Geometry check sheet. Reference: the model listing, model coordinates, mm. A direction names the side the tool comes from. Coordinates: 2 decimals unless noted, no trailing zeros. Loops run counter-clockwise (first coordinate to the right, second up) from the corner with the lowest first, then second, coordinate; pieces in that order, holes last. Notation, with made-up numbers: M -28,-32.75 L -15,-32.75 A17 cw -15,-9.75 Z; hole C 43.25,17 d5. An arc over 180 degrees is marked long. One line per question, with ' | ' between items. Start each with the question number.
from build123d import *

# Parameters (mm, degrees)
SKETCH1_R           = 3.625
SKETCH1_R_2         = 2.075
BOSS_EXTRUDE1_DEPTH = 2.41
SKETCH2_R           = 1
SKETCH2_R_2         = 0.5
BOSS_EXTRUDE3_DEPTH = 1.89
BOSS_EXTRUDE4_START = 4.3
SKETCH1_2_R         = 3.625
SKETCH1_2_R_2       = 2.075
BOSS_EXTRUDE4_DEPTH = 0.8
SKETCH3_R           = 1.5875
CUT_EXTRUDE1_DEPTH  = 18.958844524


with BuildPart() as part:
    # Sketch1 → Boss-Extrude1 (new body)
    with BuildSketch(Plane(origin=(0, 0, 0), x_dir=(1, 0, 0), z_dir=(0, 1, 0))):
        with Locations(Location((0, 0, 0), (0, 0, 270))):
            Circle(SKETCH1_R)
        with Locations(Location((0, 0, 0), (0, 0, 270))):
            Circle(SKETCH1_R_2, mode=Mode.SUBTRACT)
    extrude(amount=BOSS_EXTRUDE1_DEPTH)

    # Sketch2 → Boss-Extrude3 (add)
    with BuildSketch(Plane(origin=(0, 2.41, 0), x_dir=(1, 0, 0), z_dir=(0, 1, 0))):
        with BuildLine():
            Line((-10.6054557, -10.267177528), (-3.625, 0))
            ThreePointArc((-3.625, 0), (2.238819707, 2.851019347), (0.859585555, -3.521610097))
            Line((0.859585555, -3.521610097), (-7.459503317, -12.737599274))
            ThreePointArc((-7.459503317, -12.737599274), (-10.267690381, -13.075364593), (-10.6054557, -10.267177528))
        make_face()
        with Locations(Location((0, 0, 0), (0, 0, 270))):
            Circle(SKETCH2_R, mode=Mode.SUBTRACT)
        with Locations(Location((-9.032479508, -11.502388401, 0), (0, 0, 270))):
            Circle(SKETCH2_R_2, mode=Mode.SUBTRACT)
        with Locations(Location((-7.797268635, -9.92941221, 0), (0, 0, 270))):
            Circle(SKETCH2_R_2, mode=Mode.SUBTRACT)
        with Locations(Location((-6.562057762, -8.356436018, 0), (0, 0, 270))):
            Circle(SKETCH2_R_2, mode=Mode.SUBTRACT)
        with Locations(Location((-5.32684689, -6.783459826, 0), (0, 0, 270))):
            Circle(SKETCH2_R_2, mode=Mode.SUBTRACT)
        with Locations(Location((-4.091636017, -5.210483635, 0), (0, 0, 270))):
            Circle(SKETCH2_R_2, mode=Mode.SUBTRACT)
        with Locations(Location((-2.856425144, -3.637507443, 0), (0, 0, 270))):
            Circle(SKETCH2_R_2, mode=Mode.SUBTRACT)
    extrude(amount=BOSS_EXTRUDE3_DEPTH)

    # Sketch1<2> → Boss-Extrude4 (add)
    with BuildSketch(Plane(origin=(0, 0, 0), x_dir=(1, 0, 0), z_dir=(0, 1, 0)).offset(BOSS_EXTRUDE4_START)):
        with Locations(Location((0, 0, 0), (0, 0, 270))):
            Circle(SKETCH1_2_R)
        with Locations(Location((0, 0, 0), (0, 0, 270))):
            Circle(SKETCH1_2_R_2, mode=Mode.SUBTRACT)
    extrude(amount=BOSS_EXTRUDE4_DEPTH)

    # Sketch3 → Cut-Extrude1 (cut, through all)
    with BuildSketch(Plane(origin=(0, 4.3, 0), x_dir=(1, 0, 0), z_dir=(0, 1, 0))):
        with Locations((-8.245032577, -10.499616079)):
            Circle(SKETCH3_R)
        with Locations((-4.323238055, -5.505416671)):
            Circle(SKETCH3_R)
    extrude(amount=-CUT_EXTRUDE1_DEPTH, mode=Mode.SUBTRACT)


solid = part.part
1. Sectioned sample at B-B (y = 3.8). State how many separate pieces and enclosed holes the cut face has, and give its area (3 significant figures).
2. Sectioned sample at A-A (x = -8). Record the cut outline in (y, z), and give its area (3 significant figures).
3. Sectioned sample at D-D (y = 0.75). Record the cut outline in (x, z) (3 decimals).
4. Thickness scan on line 1 (X direction, y = 3.25, z = 0) (3 decimals); line 2 (Y direction, x = -10, z = 12.75); line 3 (X direction, y = 4.55, z = -1). Record the ranges inside material, lowest first.
5. Draft check along Z on faces 1 (the flat face through (-3.242, 3.342, 8.065)), 2 (the cylindrical face through (-2.83, 3.34, 3.14)), 3 (the flat face through (-6, 2.41, 7)). Enter one of: +Z half, -Z half, draft (parallel to the pull), parting line (faces both ways), or undercut.
6. Tool access check on faces 4 (the cylindrical face through (-1.26, 4.69, -1.65)), 5 (the cylindrical face through (-1.26, 1.19, -1.65)), 6 (the cylindrical face through (-7.22, 3.37, 9.29)). Record the directions out of +Z, -Z, +X, -X, +Y, -Y that give a thin tool (end or side, any length) a straight path to the whole face; none if there is none.
7. Sectioned sample at C-C (z = 4.75). Record the cut outline in (x, y), and give its area (3 significant figures).
8. Depth check by flat-ended pin: pin 1 Ø5 at (x, z) = (0, 0) entering from -Y; pin 2 Ø1 at (y, z) = (4, 10) entering from +X; pin 3 Ø1.2 at (x, z) = (0, 0) entering from +Y; pin 4 Ø5 at (x, z) = (-4.32, 5.51) entering from -Y. Enter the tip coordinate at first touch or a pass-through.
Result:
1) separate pieces: 1 | enclosed holes: 5 | area: 81.0 mm2
2) outline: M 2.41,6.43 L 4.3,6.43 L 4.3,8.93 L 2.41,8.93 Z; M 2.41,12.07 L 4.3,12.07 L 4.3,13.22 L 2.41,13.22 Z | area: 6.89 mm2
3) outline: C 0,0 d7.25; hole C 0,0 d4.15
4) line 1: x = -3.625 to -1, 1 to 3.625 | line 2: y = 2.41 to 4.3 | line 3: x = -3.48 to -1.82, 1.82 to 3.48
5) face 1: +Z half | face 2: undercut | face 3: draft
6) face 4: +Y | face 5: -Y | face 6: +Y, -Y
7) outline: M -6.85,2.41 L -5.72,2.41 L -5.72,4.3 L -6.85,4.3 Z; M -2.93,2.41 L -0.25,2.41 L -0.25,4.3 L -2.93,4.3 Z | area: 7.21 mm2
8) pin 1: stops at y = 0 | pin 2: stops at x = -4.54 | pin 3: passes through | pin 4: stops at y = 2.41
